Can you work these out from the drawing? Everything is in mm from the part's minimum corner. Coordinates: 2 decimals unless noted, no trailing zeros. Order: outer loops, then holes, each group sorted by start corner. A loop starts at its lowest first (then second) coordinate and runs counter-clockwise, first axis right, second up. Notation, with made-up numbers: (41, -6) - (69, -6) arc R10 cw to (69, 2) - close; hole circle Ø2 at (75.25, -5). An arc over 180 degrees is marked (long way). Use a Markdown table: item, result. Add a question column.
(1) I want a section at C-C (y = 68.5). List the corners of the cut face in (x, z) for me, and give its area (3 significant figures).
(2) For pin 1 Ø7 at (x, y) = (58.98, 51.76) entering from -Z; pin 2 Ø1 at (y, z) = (14, 3) entering from +X; pin 3 Ø1.5 at (y, z) = (43, 2) entering from -X; pin 4 Ø5 at (x, y) = (58.98, 91.06) entering from -Z, each with a flat end and sliding along its axis, tell me the tip position at first contact or that it passes through.
(3) I want a section at B-B (x = 60). List the corners of the cut face in (y, z) for me (1 decimal).
(4) I want a section at D-D (y = 47). List the corners of the cut face in (x, z) for me.
(5) If I drill on L1, parallel to Y at x = 59, z = 2.4; L2, parallel to Y at x = 52, z = 3.2; L3, parallel to Y at x = 41, z = 3.3, over which ranges is the centre line in solid material (lowest first)? Write a range as [from, to].
(6) I want a section at A-A (z = 2.65). State how many separate pieces and enclosed holes the cut face has, and give its area (3 significant figures).
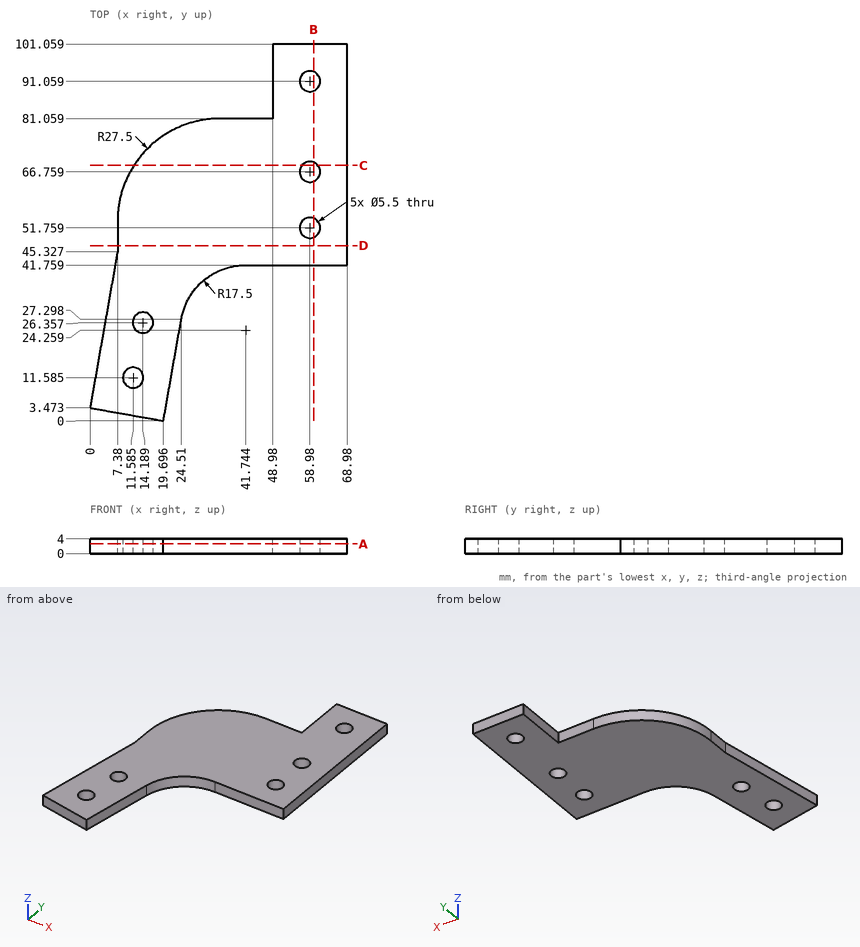
Answers follow:
| question | item | result |
|---|---|---|
| 1 | outline | (11.79, 0) - (56.85, 0) - (56.85, 4) - (11.79, 4) - close; (61.11, 0) - (68.98, 0) - (68.98, 4) - (61.11, 4) - close |
| 1 | area | 212 mm² |
| 2 | pin 1 | stops at z = 0 |
| 2 | pin 2 | stops at x = 22.25 |
| 2 | pin 3 | stops at x = 6.84 |
| 2 | pin 4 | passes through |
| 3 | outline | (41.8, 0) - (49.2, 0) - (49.2, 4) - (41.8, 4) - close; (54.3, 0) - (64.2, 0) - (64.2, 4) - (54.3, 4) - close; (69.3, 0) - (88.5, 0) - (88.5, 4) - (69.3, 4) - close; (93.6, 0) - (101.1, 0) - (101.1, 4) - (93.6, 4) - close |
| 4 | outline | (7.38, 0) - (68.98, 0) - (68.98, 4) - (7.38, 4) - close |
| 5 | L1 | y = [41.76, 49.01], [54.51, 64.01], [69.51, 88.31], [93.81, 101.06] |
| 5 | L2 | y = [41.76, 101.06] |
| 5 | L3 | y = [41.74, 81.06] |
| 6 | separate pieces | 1 |
| 6 | enclosed holes | 5 |
| 6 | area | 3,400 mm² |
